Verification items for this drawing (mm, ordinates from the low corner). Give positions to 0.01 mm unless a question says otherwise; leave off trailing zeros. Write each loop counter-clockwise with the first axis right and the second up, starting at its lowest first coordinate (ties: lowest second). Pieces come first, ordered by that corner, then holes. Notation, with made-up numbers: (44.25, 61.25) -> (75.25, 61.25) arc R10 ccw to (75.25, 66.25) -> close; hole circle Ø4 at (29, -16.75). An arc over 180 degrees is marked (long way). Answer as a JSON object with one key per item and string values.
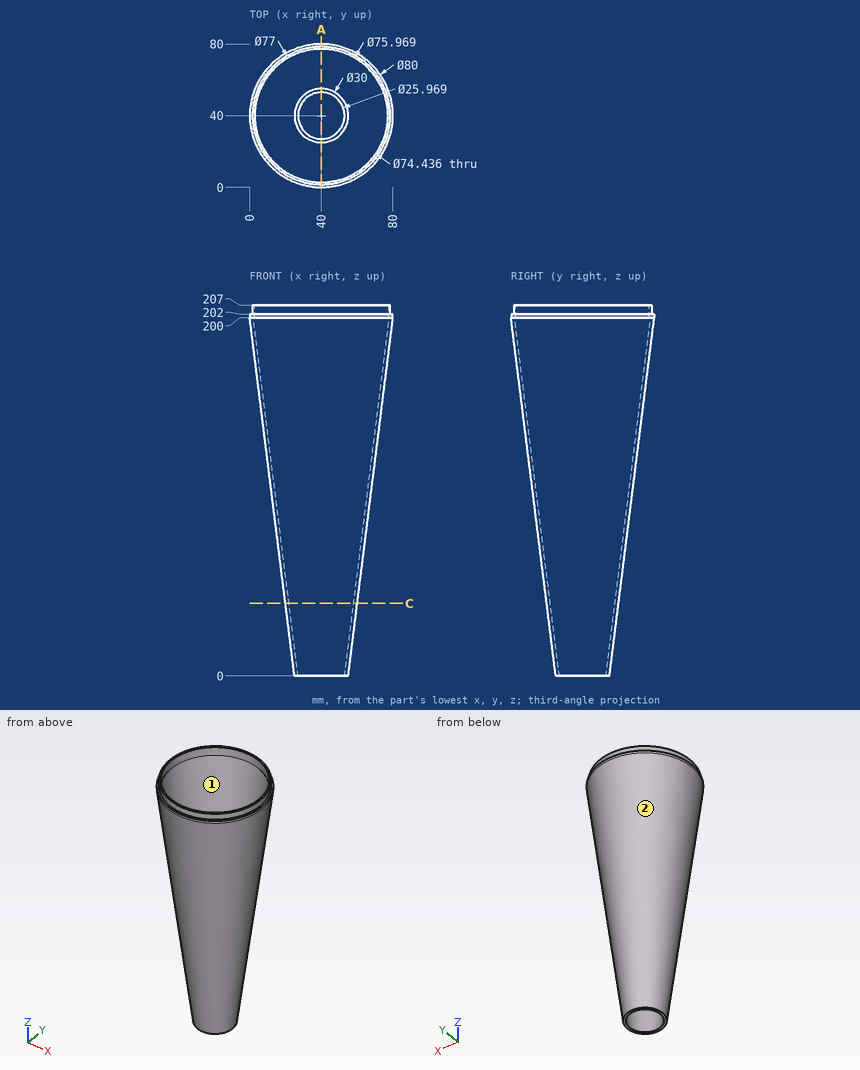
1. Sectioned sample at A-A, the plane x = 40. Enter the section's corners in (y, z).
Determined:
{"outline": "(0, 200) -> (25, 0) -> (27.02, 0) -> (2.02, 200) -> (2.78, 200) -> (2.78, 207) -> (1.5, 207) -> (1.5, 202) -> (0, 202) -> close; (52.98, 0) -> (55, 0) -> (80, 200) -> (80, 202) -> (78.5, 202) -> (78.5, 207) -> (77.22, 207) -> (77.22, 200) -> (77.98, 200) -> close"}
2. Mould release check, pull along X, two halves, no side actions. Record for the marked faces 1 and 2: released by +X, released by -X, zero draft, split by the parting line, or undercut.
Determined:
{"face 1": "undercut", "face 2": "split by the parting line"}
3. Scan lines: L1, parallel to Y at x = 40, z = 204.5; L2, parallel to Y at x = 38.5, z = 198 (1 decimal); L3, parallel to X at y = 42, z = 131. Record each from-to range of solid material in increasing order. Write a range as [from, to].
Determined:
{"L1": "[1.5, 2.78], [77.22, 78.5]", "L2": "[0.3, 2.3], [77.7, 79.7]", "L3": "[8.69, 10.71], [69.29, 71.31]"}
4. Go/stop test with flat-tipped pins: P1, Ø3, axis at y = 52, z = 128.5, coming from the +X side; P2, Ø5, axis at x = 37, z = 67, coming from the +Y side; P3, Ø4, axis at x = 44.5, y = 48.5, coming from the +Z side; P4, Ø10, axis at x = 56, z = 171, coming from the -Y side. Record where each tip stops, or that it passes through.
Determined:
{"P1": "x = 69.27", "P2": "y = 63.58", "P3": "through", "P4": "y = 5.2"}
5. Sectioned sample at C-C, the plane z = 40.5. Enter the section's corners in (x, y) (1 decimal), plus the area to 3 significant figures.
Determined:
{"outline": "circle Ø40.1 at (40, 40); hole circle Ø36.1 at (40, 40)", "area": "241 mm^2"}
